from build123d import *

# Parameters (mm, degrees)
SKETCH1_R           = 9
BOSS_EXTRUDE1_DEPTH = 21
SHELL1_T            = -4
MOVE_FACE1_BY       = 1
SKETCH1_4_R         = 9
CUT_EXTRUDE1_DEPTH  = 117.468879964
SKETCH2_R           = 9
BOSS_EXTRUDE2_DEPTH = 2


with BuildPart() as part:
    # Sketch1 → Boss-Extrude1 (new body)
    # profile 1 of 6: a face of its own
    with BuildSketch(Plane(origin=(0, 0, 0), x_dir=(1, 0, 0), z_dir=(0, 1, 0))):
        with BuildLine():
            ThreePointArc((-82, 75), (-80.535533906, 78.535533906), (-77, 80))
            Line((-77, 80), (77, 80))
            ThreePointArc((77, 80), (80.535533906, 78.535533906), (82, 75))
            Line((82, 75), (82, -75))
            ThreePointArc((82, -75), (80.535533906, -78.535533906), (77, -80))
            Line((77, -80), (-77, -80))
            ThreePointArc((-77, -80), (-80.535533906, -78.535533906), (-82, -75))
            Line((-82, -75), (-82, 75))
        make_face()
        Circle(SKETCH1_R, mode=Mode.SUBTRACT)
        with BuildLine():
            Line((-54.889206332, 64.727033293), (-26.973710346, 37.492403062))
            ThreePointArc((-26.973710346, 37.492403062), (-26.834045575, 26.179556659), (-38.146891979, 26.039891888))
            Line((-38.146891979, 26.039891888), (-66.062387966, 53.274522119))
            ThreePointArc((-66.062387966, 53.274522119), (-66.202052736, 64.587368523), (-54.889206332, 64.727033293))
        make_face(mode=Mode.SUBTRACT)
        with BuildLine():
            Line((53.274522119, 66.062387966), (26.039891888, 38.146891979))
            ThreePointArc((26.039891888, 38.146891979), (26.179556659, 26.834045575), (37.492403062, 26.973710346))
            Line((37.492403062, 26.973710346), (64.727033293, 54.889206332))
            ThreePointArc((64.727033293, 54.889206332), (64.587368523, 66.202052736), (53.274522119, 66.062387966))
        make_face(mode=Mode.SUBTRACT)
        with BuildLine():
            Line((66.062387966, -53.274522119), (38.146891979, -26.039891888))
            ThreePointArc((38.146891979, -26.039891888), (26.834045575, -26.179556659), (26.973710346, -37.492403062))
            Line((26.973710346, -37.492403062), (54.889206332, -64.727033293))
            ThreePointArc((54.889206332, -64.727033293), (66.202052736, -64.587368523), (66.062387966, -53.274522119))
        make_face(mode=Mode.SUBTRACT)
        with BuildLine():
            Line((-53.274522119, -66.062387966), (-26.039891888, -38.146891979))
            ThreePointArc((-26.039891888, -38.146891979), (-26.179556659, -26.834045575), (-37.492403062, -26.973710346))
            Line((-37.492403062, -26.973710346), (-64.727033293, -54.889206332))
            ThreePointArc((-64.727033293, -54.889206332), (-64.587368523, -66.202052736), (-53.274522119, -66.062387966))
        make_face(mode=Mode.SUBTRACT)
    # profile 2 of 6: a face of its own
    with BuildSketch(Plane(origin=(0, 0, 0), x_dir=(1, 0, 0), z_dir=(0, 1, 0))):
        with BuildLine():
            ThreePointArc((-26.973710346, 37.492403062), (-26.834045575, 26.179556659), (-38.146891979, 26.039891888))
            Line((-38.146891979, 26.039891888), (-66.062387966, 53.274522119))
            ThreePointArc((-66.062387966, 53.274522119), (-66.202052736, 64.587368523), (-54.889206332, 64.727033293))
            Line((-54.889206332, 64.727033293), (-26.973710346, 37.492403062))
        make_face()
    # profile 3 of 6: a face of its own
    with BuildSketch(Plane(origin=(0, 0, 0), x_dir=(1, 0, 0), z_dir=(0, 1, 0))):
        with BuildLine():
            ThreePointArc((-53.274522119, -66.062387966), (-64.587368523, -66.202052736), (-64.727033293, -54.889206332))
            Line((-64.727033293, -54.889206332), (-37.492403062, -26.973710346))
            ThreePointArc((-37.492403062, -26.973710346), (-26.179556659, -26.834045575), (-26.039891888, -38.146891979))
            Line((-26.039891888, -38.146891979), (-53.274522119, -66.062387966))
        make_face()
    # profile 4 of 6: a face of its own
    with BuildSketch(Plane(origin=(0, 0, 0), x_dir=(1, 0, 0), z_dir=(0, 1, 0))):
        Circle(SKETCH1_R)
    # profile 5 of 6: a face of its own
    with BuildSketch(Plane(origin=(0, 0, 0), x_dir=(1, 0, 0), z_dir=(0, 1, 0))):
        with BuildLine():
            ThreePointArc((66.062387966, -53.274522119), (66.202052736, -64.587368523), (54.889206332, -64.727033293))
            Line((54.889206332, -64.727033293), (26.973710346, -37.492403062))
            ThreePointArc((26.973710346, -37.492403062), (26.834045575, -26.179556659), (38.146891979, -26.039891888))
            Line((38.146891979, -26.039891888), (66.062387966, -53.274522119))
        make_face()
    # profile 6 of 6: a face of its own
    with BuildSketch(Plane(origin=(0, 0, 0), x_dir=(1, 0, 0), z_dir=(0, 1, 0))):
        with BuildLine():
            ThreePointArc((53.274522119, 66.062387966), (64.587368523, 66.202052736), (64.727033293, 54.889206332))
            Line((64.727033293, 54.889206332), (37.492403062, 26.973710346))
            ThreePointArc((37.492403062, 26.973710346), (26.179556659, 26.834045575), (26.039891888, 38.146891979))
            Line((26.039891888, 38.146891979), (53.274522119, 66.062387966))
        make_face()
    extrude(amount=-BOSS_EXTRUDE1_DEPTH)

    # Shell1
    shell1_openings = [part.faces().sort_by_distance(p)[0] for p in [
        (0, -21, 0),
    ]]
    offset(amount=SHELL1_T, openings=shell1_openings, kind=Kind.INTERSECTION)

    # Move Face1: a face moved inward by 1.0
    extrude(part.faces().sort_by_distance((0, -4, 0))[0], amount=MOVE_FACE1_BY, dir=(0, 1, 0), mode=Mode.SUBTRACT)

    # Sketch1<4> → Cut-Extrude1 (cut, through all)
    with BuildSketch(Plane(origin=(0, 0, 0), x_dir=(1, 0, 0), z_dir=(0, 1, 0))):
        with BuildLine():
            ThreePointArc((-26.973710346, 37.492403062), (-26.834045575, 26.179556659), (-38.146891979, 26.039891888))
            Line((-38.146891979, 26.039891888), (-66.062387966, 53.274522119))
            ThreePointArc((-66.062387966, 53.274522119), (-66.202052736, 64.587368523), (-54.889206332, 64.727033293))
            Line((-54.889206332, 64.727033293), (-26.973710346, 37.492403062))
        make_face()
        with BuildLine():
            ThreePointArc((-53.274522119, -66.062387966), (-64.587368523, -66.202052736), (-64.727033293, -54.889206332))
            Line((-64.727033293, -54.889206332), (-37.492403062, -26.973710346))
            ThreePointArc((-37.492403062, -26.973710346), (-26.179556659, -26.834045575), (-26.039891888, -38.146891979))
            Line((-26.039891888, -38.146891979), (-53.274522119, -66.062387966))
        make_face()
        with BuildLine():
            ThreePointArc((66.062387966, -53.274522119), (66.202052736, -64.587368523), (54.889206332, -64.727033293))
            Line((54.889206332, -64.727033293), (26.973710346, -37.492403062))
            ThreePointArc((26.973710346, -37.492403062), (26.834045575, -26.179556659), (38.146891979, -26.039891888))
            Line((38.146891979, -26.039891888), (66.062387966, -53.274522119))
        make_face()
        with BuildLine():
            ThreePointArc((53.274522119, 66.062387966), (64.587368523, 66.202052736), (64.727033293, 54.889206332))
            Line((64.727033293, 54.889206332), (37.492403062, 26.973710346))
            ThreePointArc((37.492403062, 26.973710346), (26.179556659, 26.834045575), (26.039891888, 38.146891979))
            Line((26.039891888, 38.146891979), (53.274522119, 66.062387966))
        make_face()
        with Locations(Location((0, 0, 0), (0, 0, 270))):
            Circle(SKETCH1_4_R)
    extrude(amount=-CUT_EXTRUDE1_DEPTH, mode=Mode.SUBTRACT)

    # Sketch2 → Boss-Extrude2 (add)
    with BuildSketch(Plane.XZ.offset(3)):
        with BuildLine():
            Line((-5.774661215, 11.647029143), (-21.002387182, 27.255448258))
            ThreePointArc((-21.002387182, 27.255448258), (-19.914815745, 34.443366807), (-23.176764095, 40.940187387))
            Line((-23.176764095, 40.940187387), (-50.411394326, 68.855683374))
            ThreePointArc((-50.411394326, 68.855683374), (-67.380663931, 69.06518053), (-67.590161087, 52.095910924))
            Line((-67.590161087, 52.095910924), (-40.355530856, 24.180414937))
            ThreePointArc((-40.355530856, 24.180414937), (-33.94122007, 20.759069904), (-26.728642769, 21.668857441))
            Line((-26.728642769, 21.668857441), (-11.500916802, 6.060438326))
            ThreePointArc((-11.500916802, 6.060438326), (-12.999009411, 0.160481598), (-11.647029143, -5.774661215))
            Line((-11.647029143, -5.774661215), (-27.255448258, -21.002387182))
            ThreePointArc((-27.255448258, -21.002387182), (-34.443366807, -19.914815745), (-40.940187387, -23.176764095))
            Line((-40.940187387, -23.176764095), (-68.855683374, -50.411394326))
            ThreePointArc((-68.855683374, -50.411394326), (-69.06518053, -67.380663931), (-52.095910924, -67.590161087))
            Line((-52.095910924, -67.590161087), (-24.180414937, -40.355530856))
            ThreePointArc((-24.180414937, -40.355530856), (-20.759069904, -33.94122007), (-21.668857441, -26.728642769))
            Line((-21.668857441, -26.728642769), (-6.060438326, -11.500916802))
            ThreePointArc((-6.060438326, -11.500916802), (-0.160481598, -12.999009411), (5.774661215, -11.647029143))
            Line((5.774661215, -11.647029143), (21.002387182, -27.255448258))
            ThreePointArc((21.002387182, -27.255448258), (19.914815745, -34.443366807), (23.176764095, -40.940187387))
            Line((23.176764095, -40.940187387), (50.411394326, -68.855683374))
            ThreePointArc((50.411394326, -68.855683374), (67.380663931, -69.06518053), (67.590161087, -52.095910924))
            Line((67.590161087, -52.095910924), (40.355530856, -24.180414937))
            ThreePointArc((40.355530856, -24.180414937), (33.94122007, -20.759069904), (26.728642769, -21.668857441))
            Line((26.728642769, -21.668857441), (11.500916802, -6.060438326))
            ThreePointArc((11.500916802, -6.060438326), (12.999009411, -0.160481598), (11.647029143, 5.774661215))
            Line((11.647029143, 5.774661215), (27.255448258, 21.002387182))
            ThreePointArc((27.255448258, 21.002387182), (34.443366807, 19.914815745), (40.940187387, 23.176764095))
            Line((40.940187387, 23.176764095), (68.855683374, 50.411394326))
            ThreePointArc((68.855683374, 50.411394326), (69.06518053, 67.380663931), (52.095910924, 67.590161087))
            Line((52.095910924, 67.590161087), (24.180414937, 40.355530856))
            ThreePointArc((24.180414937, 40.355530856), (20.759069904, 33.94122007), (21.668857441, 26.728642769))
            Line((21.668857441, 26.728642769), (6.060438326, 11.500916802))
            ThreePointArc((6.060438326, 11.500916802), (0.160481598, 12.999009411), (-5.774661215, 11.647029143))
        make_face()
        with BuildLine():
            ThreePointArc((-54.889206332, -64.727033293), (-66.202052736, -64.587368523), (-66.062387966, -53.274522119))
            Line((-66.062387966, -53.274522119), (-38.146891979, -26.039891888))
            ThreePointArc((-38.146891979, -26.039891888), (-26.834045575, -26.179556659), (-26.973710346, -37.492403062))
            Line((-26.973710346, -37.492403062), (-54.889206332, -64.727033293))
        make_face(mode=Mode.SUBTRACT)
        with Locations(Location((0, 0, 0), (0, 0, 90))):
            Circle(SKETCH2_R, mode=Mode.SUBTRACT)
        with BuildLine():
            Line((-53.274522119, 66.062387966), (-26.039891888, 38.146891979))
            ThreePointArc((-26.039891888, 38.146891979), (-26.179556659, 26.834045575), (-37.492403062, 26.973710346))
            Line((-37.492403062, 26.973710346), (-64.727033293, 54.889206332))
            ThreePointArc((-64.727033293, 54.889206332), (-64.587368523, 66.202052736), (-53.274522119, 66.062387966))
        make_face(mode=Mode.SUBTRACT)
        with BuildLine():
            ThreePointArc((38.146891979, 26.039891888), (26.834045575, 26.179556659), (26.973710346, 37.492403062))
            Line((26.973710346, 37.492403062), (54.889206332, 64.727033293))
            ThreePointArc((54.889206332, 64.727033293), (66.202052736, 64.587368523), (66.062387966, 53.274522119))
            Line((66.062387966, 53.274522119), (38.146891979, 26.039891888))
        make_face(mode=Mode.SUBTRACT)
        with BuildLine():
            ThreePointArc((26.039891888, -38.146891979), (26.179556659, -26.834045575), (37.492403062, -26.973710346))
            Line((37.492403062, -26.973710346), (64.727033293, -54.889206332))
            ThreePointArc((64.727033293, -54.889206332), (64.587368523, -66.202052736), (53.274522119, -66.062387966))
            Line((53.274522119, -66.062387966), (26.039891888, -38.146891979))
        make_face(mode=Mode.SUBTRACT)
    extrude(amount=BOSS_EXTRUDE2_DEPTH)


solid = part.part
Read the model definition and answer for the solid it produces. Units are mm, in the model's axes. A direction names the side the tool comes from. Coordinates: 2 decimals unless noted, no trailing zeros. Loops run counter-clockwise (first coordinate to the right, second up) from the corner with the lowest first, then second, coordinate; pieces in that order, holes last.
Q1. Which of the six approach directions +Z, -Z, +X, -X, +Y, -Y give full straight-line access (tool end or side, diameter ignored) to faces 4 (the face through (-82, -10, 1)), 5 (the face through (-34.043, -3.986, 20.778)), 6 (the face through (52.3, -2.46, 39.85))?
Q2. The mould has two halves that part along Z. Classify faces 1 (the face through (1, 0, -19)), 2 (the face through (39.85, -2.46, -52.3)), 3 (the face through (-1, -12, -76)): +Z half, -Z half, draft (parallel to the pull), parting line (faces both ways), or undercut.
Q3. Consider probe 1 along X at (y, z) = (-3.2, 0); probe 2 along Z at (x, y) = (-50, -17); probe 3 along X at (y, z) = (-17.5, 1). Determine where each line is inside the solid, lowest interval first.
Q4. Each of these flat-tipped pins is pushed along its axis until it touches: pin 1 Ø12 at (x, z) = (-56, -50.5) entering from -Y; pin 2 Ø11 at (x, z) = (0, 0) entering from +Y. Where does it stop, or does it pass through?
Q5. The part is cut by section A-A on z = 0. Write down the section's boundary in (x, y), and give its area (3 significant figures).
Q6. The part is cut by section C-C on x = 0. Write down the section's boundary in (y, z).
Q7. The part is cut by section B-B on y = -16. Write down the section's boundary in (x, z), and give its area (3 significant figures).
Results below:
1. face 4: +Z, -Z, -X, +Y, -Y
1. face 5: -Y
1. face 6: +Y, -Y
2. face 1: draft
2. face 2: undercut
2. face 3: undercut
3. probe 1: x = -82 to -78, -13 to -9, 9 to 13, 78 to 82
3. probe 2: z = -80 to -76, 76 to 80
3. probe 3: x = -82 to -78, 78 to 82
4. pin 1: stops at y = -5
4. pin 2: passes through
5. outline: (-82, -21) - (-78, -21) - (-78, -3) - (-13, -3) - (-13, -5) - (-9, -5) - (-9, 0) - (-82, 0) - close; (9, -5) - (13, -5) - (13, -3) - (78, -3) - (78, -21) - (82, -21) - (82, 0) - (9, 0) - close
5. area: 598 mm2
6. outline: (-21, -80) - (0, -80) - (0, -9) - (-5, -9) - (-5, -13) - (-3, -13) - (-3, -76) - (-21, -76) - close; (-21, 76) - (-3, 76) - (-3, 13) - (-5, 13) - (-5, 9) - (0, 9) - (0, 80) - (-21, 80) - close
7. outline: (-82, -75) arc R5 ccw to (-77, -80) - (77, -80) arc R5 ccw to (82, -75) - (82, 75) arc R5 ccw to (77, 80) - (-77, 80) arc R5 ccw to (-82, 75) - close; hole (-78, -75) arc R1 ccw to (-77, -76) - (77, -76) arc R1 ccw to (78, -75) - (78, 75) arc R1 ccw to (77, 76) - (-77, 76) arc R1 ccw to (-78, 75) - close
7. area: 2,510 mm2
